from build123d import *

# Parameters (mm, degrees)
EXTRUSION1_DEPTH = 240
ESQUISSE2_R      = 1.5
EXTRUSION2_DEPTH = 242.541404318
ESQUISSE3_W      = 1.5
ESQUISSE3_H      = 20
EXTRUSION3_DEPTH = 20
ESQUISSE5_W      = 1.5
ESQUISSE5_H      = 20
EXTRUSION4_DEPTH = 20
ESQUISSE6_R      = 1.5
EXTRUSION5_DEPTH = 262.423506977


with BuildPart() as part:
    # Esquisse1 → Extrusion1 (new body)
    with BuildSketch(Plane.XY):
        Polygon((0, 0), (20, 0), (20, 1.5), (1.5, 1.5), (1.5, 20), (0, 20), align=None)
    extrude(amount=EXTRUSION1_DEPTH)

    # Esquisse2 → Extrusion2 (cut, through all)
    with BuildSketch(Plane(origin=(0, 1.5, 0), x_dir=(1, 0, 0), z_dir=(0, 1, 0))):
        with Locations(Location((10, -39, 0), (0, 0, 180))):
            Circle(ESQUISSE2_R)
        with Locations(Location((10, -201, 0), (0, 0, 180))):
            Circle(ESQUISSE2_R)
    extrude(amount=-EXTRUSION2_DEPTH, mode=Mode.SUBTRACT)

    # Esquisse3 → Extrusion3 (add)
    with BuildSketch(Plane.XY.offset(240)):
        with Locations((0.75, 10)):
            Rectangle(ESQUISSE3_W, ESQUISSE3_H)
    extrude(amount=EXTRUSION3_DEPTH)

    # Esquisse5 → Extrusion4 (add)
    with BuildSketch(Plane(origin=(0, 0, 0), x_dir=(-1, 0, 0), z_dir=(0, 0, -1))):
        with Locations((-0.75, 10)):
            Rectangle(ESQUISSE5_W, ESQUISSE5_H)
    extrude(amount=EXTRUSION4_DEPTH)

    # Esquisse6 → Extrusion5 (cut, through all)
    with BuildSketch(Plane(origin=(1.5, 0, 0), x_dir=(0, 0, -1), z_dir=(1, 0, 0))):
        with Locations(Location((-248.5, 10, 0), (0, 0, 90))):
            Circle(ESQUISSE6_R)
        with Locations(Location((8.5, 10, 0), (0, 0, 90))):
            Circle(ESQUISSE6_R)
        with Locations(Location((-181, 10, 0), (0, 0, 90))):
            Circle(ESQUISSE6_R)
        with Locations(Location((-59, 10, 0), (0, 0, 90))):
            Circle(ESQUISSE6_R)
    extrude(amount=-EXTRUSION5_DEPTH, mode=Mode.SUBTRACT)


solid = part.part
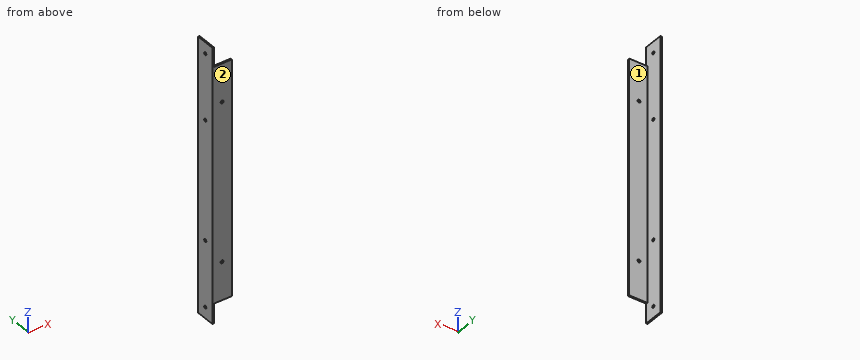
Build history of the part. All positions in model axes, mm. Face numbers are marked on the shaded views. Give positions to 0.01 mm unless a question says otherwise; leave off trailing zeros. Write each loop counter-clockwise with the first axis right and the second up, starting at its lowest first coordinate (ties: lowest second). Pieces come first, ordered by that corner, then holes. Notation, with made-up numbers: (-17.5, 49) - (18.5, 49) arc R17 cw to (18.5, 75) - close; hole circle Ø5 at (33.25, 89). An arc over 180 degrees is marked (long way). Use one line per item in the form item = value. Start each with the question number.
1. Band-saw the part on B-B on x = 15. Write the cut outline in (y, z), plus the area to 3 significant figures.
2. Drop flat-ended pins along their axis: pin 1 Ø4 at (y, z) = (11.5, 105.5) entering from -X; pin 2 Ø12 at (x, y) = (15.5, 10) entering from -Z; pin 3 Ø10 at (y, z) = (13.5, 132) entering from +X; pin 4 Ø1.6 at (x, y) = (11.5, 1) entering from +Z. Give the stop position or say it passes through.
3. Probe line 1 (Z direction, x = 0.7, y = 10); line 2 (Z direction, x = 10, y = 0.6); line 3 (X direction, y = 0.8, z = 201). List the from-to ranges inside material, lowest first. Write a range as [from, to].
4. Two-plate mould, pull along Y, no slides. Class the marked faces 1 and 2: released by +Y, released by -Y, zero draft, split by the parting line, or undercut.
5. Band-saw the part on A-A on z = 82. Write the cut outline in (x, y), plus the area to 4 significant figures.
6. Band-saw the part on C-C on y = 17. Write the cut outline in (x, z), plus the area to 3 significant figures.
Conclusion:
q1.outline = (0, 0) - (1.5, 0) - (1.5, 240) - (0, 240) - close
q1.area = 360 mm²
q2.pin_1 = 0
q2.pin_2 = through
q2.pin_3 = 1.5
q2.pin_4 = 240
q3.line_1 = [-20, -10], [-7, 57.5], [60.5, 179.5], [182.5, 247], [250, 260]
q3.line_2 = [0, 37.5], [40.5, 199.5], [202.5, 240]
q3.line_3 = [0, 8.5], [11.5, 20]
q4.face_1 = released by +Y
q4.face_2 = released by -Y
q5.outline = (0, 0) - (20, 0) - (20, 1.5) - (1.5, 1.5) - (1.5, 20) - (0, 20) - close
q5.area = 57.75 mm²
q6.outline = (0, -20) - (1.5, -20) - (1.5, 260) - (0, 260) - close
q6.area = 420 mm²
